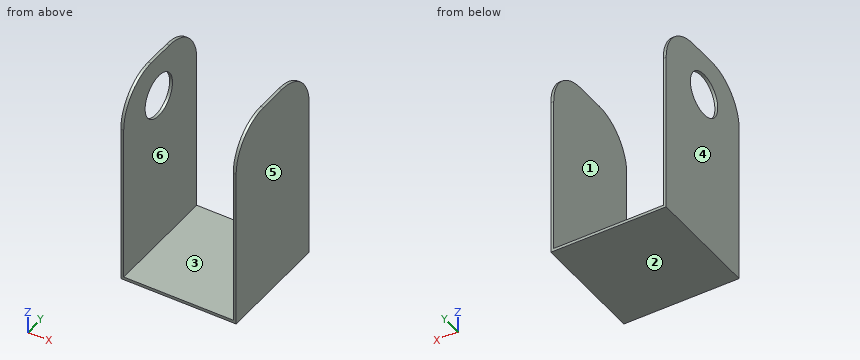
from build123d import *

# Parameters (mm, degrees)
F0_W     = 50.8
F0_H     = 50.8
F1_DEPTH = 1.27
F2_W     = 1.27
F2_H     = 50.8
F3_DEPTH = 88.9
F4_R     = 19.05
F5_R     = 19.05
F7_D     = 19.05
F7_DEPTH = 1.271


with BuildPart() as f1:
    # F0 (on Top) → F1 (new body)
    with BuildSketch(Plane.XY):
        with Locations((3.9132147372, 0.9917675793)):
            Rectangle(F0_W, F0_H)
    extrude(amount=F1_DEPTH)

    # F2 (on face) → F3 (join)
    with BuildSketch(Plane.XY.offset(1.27)):
        with Locations((-20.8517852628, 0.9917675793)):
            Rectangle(F2_W, F2_H)
        with Locations((28.6782147372, 0.9917675793)):
            Rectangle(F2_W, F2_H)
    extrude(amount=F3_DEPTH)

    # F4
    f4_edges = [f1.edges().sort_by_distance(p)[0] for p in [
        (28.678215, 26.391768, 90.17),
        (-20.851785, 26.391768, 90.17),
    ]]
    fillet(f4_edges, radius=F4_R)

    # F5
    f5_edges = [f1.edges().sort_by_distance(p)[0] for p in [
        (-20.851785, -24.408232, 90.17),
        (28.678215, -24.408232, 90.17),
    ]]
    fillet(f5_edges, radius=F5_R)

    # F7 (through all, one way)
    with BuildSketch(Plane.YZ.offset(-20.2167852628)):
        with Locations((0, 71.12)):
            Circle(F7_D / 2)
    extrude(amount=-F7_DEPTH, mode=Mode.SUBTRACT)


solid = f1.part
Can you work these out from the model? Positions are in its coordinate system, mm. Face numbers are marked on the shaded views. A direction names the side the tool comes from. Round coordinates to 2 decimals unless told otherwise and drop trailing zeros. Loops run counter-clockwise (first coordinate to the right, second up) from the corner with the lowest first, then second, coordinate; pieces in that order, holes last. Notation, with made-up numbers: (17, -39.5) - (46, -39.5) arc R19 ccw to (46, -30.5) - close; hole circle Ø8 at (1.5, -15.5). An arc over 180 degrees is marked (long way). Use CSV: the item, a comma, the result in double quotes. Start each with the question number.
1) We'd pull the mould along X, two halves only. Please class the marked faces 1, 2, 3 and 4: released by +X, released by -X, zero draft, split by the parting line, or undercut.
2) Please list where these lines run through material, in increasing order: probe 1 along X at (y, z) = (22.5, 61); probe 2 along Y at (x, z) = (-21, 71); probe 3 along Z at (x, y) = (-20.8, 0) (3 decimals). Write a range as [from, to].
3) If we section it at A-A on y = 0: Write out the boundary of the cut face in (x, z) (3 decimals), plus the area to 3 significant figures.
4) If we section it at C-C on z = 79: Write out the boundary of the cut face in (x, y), plus the area to 3 significant figures.
5) If we section it at B-B on z = 31: Write out the boundary of the cut face in (x, y).
6) If we section it at D-D on x = 2.5: Write out the boundary of the cut face in (y, z).
7) For pin 1 Ø10 at (x, z) = (21.5, 28) entering from -Y; pin 2 Ø2 at (x, y) = (13, 11.5) entering from +Z, each with a flat end and sliding along its axis, tell me the tip position at first contact or that it passes through.
8) For the marked faces 5 and 6, which set-ups out of +Z, -Z, +X, -X, +Y, -Y let a thin tool reach every point of the face, with its end or its side?
Geometry results:
1,face 1,"undercut"
1,face 2,"zero draft"
1,face 3,"undercut"
1,face 4,"released by -X"
2,probe 1,"x = [-21.49, -20.22], [28.04, 29.31]"
2,probe 2,"y = [-24.41, -9.52], [9.52, 26.39]"
2,probe 3,"z = [0, 61.595], [80.645, 90.17]"
3,outline,"(-21.487, 0) - (29.313, 0) - (29.313, 90.17) - (28.043, 90.17) - (28.043, 1.27) - (-20.217, 1.27) - (-20.217, 61.595) - (-21.487, 61.595) - close; (-21.487, 80.645) - (-20.217, 80.645) - (-20.217, 90.17) - (-21.487, 90.17) - close"
3,area,"266 mm2"
4,outline,"(-21.49, -22.7) - (-20.22, -22.7) - (-20.22, -5.35) - (-21.49, -5.35) - close; (-21.49, 5.35) - (-20.22, 5.35) - (-20.22, 24.69) - (-21.49, 24.69) - close; (28.04, -22.7) - (29.31, -22.7) - (29.31, 24.69) - (28.04, 24.69) - close"
4,area,"107 mm2"
5,outline,"(-21.49, -24.41) - (-20.22, -24.41) - (-20.22, 26.39) - (-21.49, 26.39) - close; (28.04, -24.41) - (29.31, -24.41) - (29.31, 26.39) - (28.04, 26.39) - close"
6,outline,"(-24.41, 0) - (26.39, 0) - (26.39, 1.27) - (-24.41, 1.27) - close"
7,pin 1,"passes through"
7,pin 2,"stops at z = 1.27"
8,face 5,"+Z, -Z, +X, +Y, -Y"
8,face 6,"+Z, +Y, -Y"
